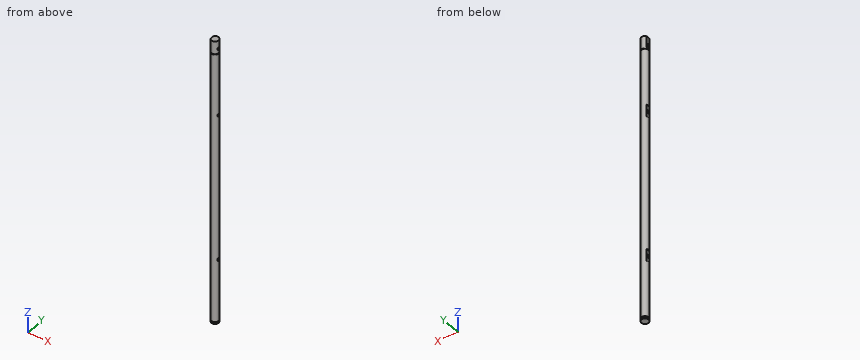
```python
from build123d import *

# Parameters (mm, degrees)
SKETCH1_R               = 3
BOSS_EXTRUDE1_DEPTH     = 235
SKETCH2_W               = 0.5
SKETCH2_H               = 0.8
SKETCH3_W               = 0.5
SKETCH3_H               = 10
SKETCH3_H_2             = 9
CUT_EXTRUDE1_DEPTH      = 10
CUT_EXTRUDE1_DEPTH_BACK = 10
M3_TAPPED_HOLE1_D       = 2.5
M3X0_5_TAPPED_HOLE1_D   = 2.5


with BuildPart() as part:
    # Sketch1 → Boss-Extrude1 (new body)
    with BuildSketch(Plane.XY):
        Circle(SKETCH1_R)
    extrude(amount=BOSS_EXTRUDE1_DEPTH)

    # Sketch2 → Cut-Revolve1 (revolve, cut)
    with BuildSketch(Plane(origin=(0, 0, 0), x_dir=(1, 0, 0), z_dir=(0, 1, 0))):
        with Locations((-2.75, -1.6)):
            Rectangle(SKETCH2_W, SKETCH2_H)
        with Locations((-2.75, -224.4)):
            Rectangle(SKETCH2_W, SKETCH2_H)
    revolve(axis=Axis((0, 0, 240), (0, 0, -1)), mode=Mode.SUBTRACT)

    # Sketch3 → Cut-Extrude1 (cut, two sides)
    with BuildSketch(Plane(origin=(0, 0, 0), x_dir=(1, 0, 0), z_dir=(0, 1, 0))) as cut_extrude1_sk:
        with Locations((-2.75, -53)):
            Rectangle(SKETCH3_W, SKETCH3_H)
        with Locations((-2.75, -173)):
            Rectangle(SKETCH3_W, SKETCH3_H)
        with Locations((-2.75, -230.5)):
            Rectangle(SKETCH3_W, SKETCH3_H_2)
    extrude(amount=CUT_EXTRUDE1_DEPTH, mode=Mode.SUBTRACT)
    extrude(cut_extrude1_sk.sketch, amount=-CUT_EXTRUDE1_DEPTH_BACK, mode=Mode.SUBTRACT)

    # M3 Tapped Hole1 (through all)
    with Locations(Plane(origin=(-2.5, 0, 173), x_dir=(0, 0, -1), z_dir=(-1, 0, 0))):
        with Locations((0, 0), (120, 0)):
            Hole(M3_TAPPED_HOLE1_D / 2)

    # M3x0.5 Tapped Hole1 (through all)
    with Locations(Plane(origin=(-2.5, 0, 228.3), x_dir=(0, 0, -1), z_dir=(-1, 0, 0))):
        with Locations((0, 0)):
            Hole(M3X0_5_TAPPED_HOLE1_D / 2)


solid = part.part
```
Read the model definition and answer for the solid it produces. Units are mm, in the model's axes. Coordinates: 2 decimals unless noted, no trailing zeros. Loops run counter-clockwise (first coordinate to the right, second up) from the corner with the lowest first, then second, coordinate; pieces in that order, holes last.
(1) Flat-ended cylindrical pins translate along their axes: pin 1 Ø3 at (x, z) = (-2, 165) entering from +Y; pin 2 Ø2 at (y, z) = (-2.5, 144) entering from +X; pin 3 Ø1 at (y, z) = (0.5, 230) entering from -X. Find the tip coordinate at first contact, or state that the pin passes through.
Solution:
pin 1: stops at y = 2.96
pin 2: stops at x = 2.6
pin 3: stops at x = -2.5
(2) The part is cut by section C-C (z = 119). Determine the outline of the cut face in (x, y).
Solution:
outline: circle Ø6 at (0, 0)
(3) The part is cut by section B-B (y = 0). Count the separate pieces of the cut face and the enclosed holes in it, and give its area (3 significant figures).
Solution:
separate pieces: 4
enclosed holes: 0
area: 1,350 mm2
(4) The part is cut by section A-A (x = 0.75). Determine the outline of the cut face in (y, z).
Solution:
outline: (-2.9, 0) - (2.9, 0) - (2.9, 1.2) - (2.38, 1.2) - (2.38, 2) - (2.9, 2) - (2.9, 224) - (2.38, 224) - (2.38, 224.8) - (2.9, 224.8) - (2.9, 235) - (-2.9, 235) - (-2.9, 224.8) - (-2.38, 224.8) - (-2.38, 224) - (-2.9, 224) - (-2.9, 2) - (-2.38, 2) - (-2.38, 1.2) - (-2.9, 1.2) - close; hole circle Ø2.5 at (0, 53); hole circle Ø2.5 at (0, 173); hole circle Ø2.5 at (0, 228.3)
(5) Consider line 1 along Z through (x, y) = (1.25, 2.5); line 2 along Y through (x, z) = (-0.3, 53); line 3 along Z through (x, y) = (1, -1). Determine where each line is inside the solid, lowest interval first.
Solution:
line 1: z = 0 to 1.2, 2 to 224, 224.8 to 235
line 2: y = -2.98 to -1.25, 1.25 to 2.98
line 3: z = 0 to 52.25, 53.75 to 172.25, 173.75 to 227.55, 229.05 to 235
